from build123d import *

# Parameters (mm, degrees)
F0_R     = 1.6375
F1_DEPTH = 6.35
F2_R     = 1.7272
F3_DEPTH = 25


with BuildPart() as f1:
    # F0 (on Top) → F1 (new body)
    with BuildSketch(Plane.XY):
        with BuildLine():
            ThreePointArc((86.602541, -50), (96.592583, -25.881904), (100, 0))
            ThreePointArc((100, 0), (96.592583, 25.881904), (86.602541, 49.999999))
            ThreePointArc((86.602541, 49.999999), (50.000001, 86.60254), (0, 100))
            ThreePointArc((0, 100), (-50.000001, 86.60254), (-86.602541, 49.999999))
            ThreePointArc((-86.602541, 49.999999), (-100, 1e-06), (-86.602542, -49.999998))
            ThreePointArc((-86.602542, -49.999998), (-50.000001, -86.60254), (0, -100))
            ThreePointArc((0, -100), (50, -86.60254), (86.602541, -50))
        make_face()
        with Locations((-78.364474, -45.24375)):
            Circle(F0_R, mode=Mode.SUBTRACT)
        with Locations((78.364474, -45.24375)):
            Circle(F0_R, mode=Mode.SUBTRACT)
        with BuildLine():
            ThreePointArc((42.64375, 73.861142), (73.861142, 42.64375), (85.2875, 0))
            ThreePointArc((85.2875, 0), (73.861142, -42.64375), (42.64375, -73.861142))
            ThreePointArc((42.64375, -73.861142), (-42.64375, -73.861142), (-85.2875, 0))
            ThreePointArc((-85.2875, 0), (-42.64375, 73.861142), (42.64375, 73.861142))
        make_face(mode=Mode.SUBTRACT)
        with Locations((0, 90.4875)):
            Circle(F0_R, mode=Mode.SUBTRACT)
        with BuildLine():
            ThreePointArc((86.602541, 49.999999), (96.592583, 25.881904), (100, 0))
            ThreePointArc((100, 0), (96.592583, -25.881904), (86.602541, -50))
            Line((86.602541, -50), (115.470054, 0))
            Line((115.470054, 0), (86.602541, 49.999999))
        make_face()
        with BuildLine():
            ThreePointArc((0, 100), (50.000001, 86.60254), (86.602541, 49.999999))
            Line((86.602541, 49.999999), (57.735027, 100))
            Line((57.735027, 100), (0, 100))
        make_face()
        with BuildLine():
            Line((57.735027, -100), (86.602541, -50))
            ThreePointArc((86.602541, -50), (50, -86.60254), (0, -100))
            Line((0, -100), (57.735027, -100))
        make_face()
        with BuildLine():
            ThreePointArc((-86.602541, 49.999999), (-50.000001, 86.60254), (0, 100))
            Line((0, 100), (-57.735027, 100))
            Line((-57.735027, 100), (-86.602541, 49.999999))
        make_face()
        with BuildLine():
            Line((-57.735027, -100), (0, -100))
            ThreePointArc((0, -100), (-50.000001, -86.60254), (-86.602542, -49.999998))
            Line((-86.602542, -49.999998), (-57.735027, -100))
        make_face()
        with BuildLine():
            ThreePointArc((-86.602542, -49.999998), (-100, 1e-06), (-86.602541, 49.999999))
            Line((-86.602541, 49.999999), (-115.470054, 0))
            Line((-115.470054, 0), (-86.602542, -49.999998))
        make_face()
    extrude(amount=F1_DEPTH)

    # F2 (on Top) → F3 (cut)
    with BuildSketch(Plane.XY):
        with Locations((38.148276, 95)):
            Circle(F2_R)
        with Locations((-38.148276, 95)):
            Circle(F2_R)
        with Locations((-63.198276, 80.537376)):
            Circle(F2_R)
        with Locations((-101.346551, 14.462624)):
            Circle(F2_R)
        with Locations((-101.346551, -14.462624)):
            Circle(F2_R)
        with Locations((-63.198276, -80.537376)):
            Circle(F2_R)
        with Locations((-38.148276, -95)):
            Circle(F2_R)
        with Locations((38.148276, -95)):
            Circle(F2_R)
        with Locations((63.198276, -80.537376)):
            Circle(F2_R)
        with Locations((101.346551, -14.462624)):
            Circle(F2_R)
        with Locations((101.346551, 14.462624)):
            Circle(F2_R)
        with Locations((63.198276, 80.537376)):
            Circle(F2_R)
    extrude(amount=F3_DEPTH, mode=Mode.SUBTRACT)


solid = f1.part
Input: part model. Units: mm. Frame: model coordinates. Round coordinates to 2 decimals unless told otherwise and drop trailing zeros. Write each loop counter-clockwise with the first axis right and the second up, starting at its lowest first coordinate (ties: lowest second). Pieces come first, ordered by that corner, then holes.
1) Ray query, L1, parallel to X at y = -44.5, z = 2.5; L2, parallel to X at y = -95, z = 2; L3, parallel to X at y = 60, z = 5.5. Return the intervals inside material, ascending.
2) Cut plane B-B (y = 65). Return the cut outline in (x, z).
3) Contact query for a flat-ended pin moving along its axis: P1, Ø2, axis at x = 0, y = 90.49, coming from the +Z side. Output: stop coordinate, or through.
4) Cut plane A-A (x = -22). Return the cut outline in (y, z).
5) Cut plane C-C (z = 3.5). Count the separate pieces of the cut face and the enclosed holes in it, then the cut area to 3 significant figures.
Geometry says:
1. L1: x = -89.78 to -79.82, -76.91 to -72.76, 72.76 to 76.91, 79.82 to 89.78
1. L2: x = -60.62 to -39.88, -36.42 to 36.42, 39.88 to 60.62
1. L3: x = -80.83 to -60.61, 60.61 to 80.83
2. outline: (-77.94, 0) - (-55.22, 0) - (-55.22, 6.35) - (-77.94, 6.35) - close; (55.22, 0) - (77.94, 0) - (77.94, 6.35) - (55.22, 6.35) - close
3. P1: passes through
4. outline: (-100, 0) - (-82.4, 0) - (-82.4, 6.35) - (-100, 6.35) - close; (82.4, 0) - (100, 0) - (100, 6.35) - (82.4, 6.35) - close
5. separate pieces: 1
5. enclosed holes: 16
5. area: 11,700 mm2
